Autodesk Inventor part; units mm, degrees
ref_plane "YZ Plane" through (0, 0, 0) normal (1, 0, 0) x (0, 1, 0)
ref_plane "XZ Plane" through (0, 0, 0) normal (0, 1, 0) x (-1, 0, 0)
ref_plane "XY Plane" through (0, 0, 0) normal (0, 0, 1) x (1, 0, 0)
sketch "Sketch1" plane through (0, 0, 0) normal (0, 0, 1) x (1, 0, 0)
  line L0 (0, 0) -> (0, 4)
  line L1 (0, 4) -> (0.36, 4)
  line L2 (0.36, 4) -> (2.36, 2)
  line L3 (2.36, 2) -> (12, 2)
  line L4 (12, 2) -> (12, 0)
  line L5 (12, 0) -> (0, 0)
  dimension "d0" = 4
  dimension "d1" = 0.36
  dimension "d2" = 135
  dimension "d3" = 12
  dimension "d4" = 2
revolve "Revolution1" add sketch "Sketch1" angle 360 about axis through (12, 0, 0) along (-1, 0, 0)
chamfer "Chamfer1" distance 0.5 angle 45 1 edges at (12, -2, 0)
sketch "Sketch2" plane through (0, 0, 0) normal (-1, 0, 0) x (0, 0, 1)
  circle A0 centre (0, 0) radius 4
  line L0 (-1.4434, 0) -> (-0.7217, 1.25)
  line L1 (-0.7217, 1.25) -> (0.7217, 1.25)
  line L2 (0.7217, 1.25) -> (1.4434, 0)
  line L3 (1.4434, 0) -> (0.7217, -1.25)
  line L4 (0.7217, -1.25) -> (-0.7217, -1.25)
  line L5 (-0.7217, -1.25) -> (-1.4434, 0)
  dimension "d9" = 2.5
extrude "Extrusion1" cut sketch "Sketch2" against normal blind 1.5 contours L0 L1 L2 L3 L4 L5
thread "Thread1"
properties part number "FHS4x12" material "Steel, Alloy"
Part model, mm, in its own coordinate system. A direction names the side the tool comes from. Coordinates: 2 decimals unless noted, no trailing zeros. Order: outer loops, then holes, each group sorted by start corner. A loop starts at its lowest first (then second) coordinate and runs counter-clockwise, first axis right, second up. Notation, with made-up numbers: M -7,-18.5 L 51,-18.5 A19 ccw 51,10.5 Z; hole C 6.5,18 d7. An arc over 180 degrees is marked long. One line per question, with ' | ' between items.
Q1. Pin check, flat tips, straight feed: P1, Ø4, axis at x = 3, z = -1.5, coming from the -Y side; P2, Ø3, axis at x = 3.5, z = -1.5, coming from the -Y side; P3, Ø0.7, axis at x = 1, z = 0, coming from the -Y side. Stop position of each tip, or through.
A:
P1: stops at y = -3.14 | P2: stops at y = -2.05 | P3: stops at y = -3.71
Q2. Drill centre lines: line 1 (Y direction, x = 2, z = -2); line 2 (X direction, y = 0, z = -1); line 3 (Z direction, x = 2.5, y = 0). Where is each one in solid material? Low to high.
A:
line 1: y = -1.25 to 1.25 | line 2: x = 1.5 to 12 | line 3: z = -2 to 2
Q3. Slice it at C-C (x = 1.75). Give the cut face in (y, z).
A:
outline: C 0,0 d5.22
Q4. 3-axis set-ups, long thin cutter, end or side, ignore diameter. For faces 1 (the face through (12, 0, 0)), 2 (the face through (7, 0, -2)), 3 (the face through (1, 1.25, 0)): which of +Z, -Z, +X, -X, +Y, -Y reach the whole face in a straight line?
A:
face 1: +Z, -Z, +X, +Y, -Y | face 2: +X | face 3: -X
Q5. Two-plate mould, pull along Z, no slides. Class faces 4 (the face through (0, 2, 0)), 5 (the face through (0.74, 0.63, 1.08)), 6 (the face through (0.183, -0.867, -3.905)): +Z half, -Z half, draft (parallel to the pull), parting line (faces both ways), or undercut.
A:
face 4: draft | face 5: undercut | face 6: parting line
Q6. Slice it at A-A (z = 0). Give the cut face in (x, y), and give its area (3 significant figures).
A:
outline: M 0,-4 L 0.36,-4 L 2.36,-2 L 11.5,-2 L 12,-1.5 L 12,1.5 L 11.5,2 L 2.36,2 L 0.36,4 L 0,4 L 0,1.25 L 1.5,1.25 L 1.5,-1.25 L 0,-1.25 Z | area: 49.4 mm^2
Q7. Slice it at B-B (x = 9.25). Give the cut face in (y, z).
A:
outline: C 0,0 d4
